```python
from build123d import *

# Parameters (mm, degrees)
SKETCH_1_R          = 2.5
EXTRUDE_1_DEPTH     = 2
SKETCH_2_R          = 1.5
EXTRUDE_2_DEPTH     = 33
FILLET_2_R          = 0.3
CUT_EXTRUDE_1_DEPTH = 1
FILLET_1_R          = 0.1


with BuildPart() as part:
    # Эскиз1 → Бобышка-Вытянуть1 (new body)
    with BuildSketch(Plane.XY):
        Circle(SKETCH_1_R)
    extrude(amount=EXTRUDE_1_DEPTH)

    # Эскиз2 → Бобышка-Вытянуть2 (add)
    with BuildSketch(Plane(origin=(0, 0, 0), x_dir=(-1, 0, 0), z_dir=(0, 0, -1))):
        Circle(SKETCH_2_R)
    extrude(amount=EXTRUDE_2_DEPTH)

    # Скругление2
    fillet_2_edges = [part.edges().sort_by_distance(p)[0] for p in [
        (-2.5, 0, 0),
        (-2.5, 0, 2),
    ]]
    fillet(fillet_2_edges, radius=FILLET_2_R)

    # Эскиз3 → Вырез-Вытянуть1 (cut)
    with BuildSketch(Plane.XY.offset(2)):
        Polygon((-0.45, 1.5), (0.45, 1.5), (0.45, 0.45), (1.5, 0.45), (1.5, -0.45), (0.45, -0.45), (0.45, -1.5), (-0.45, -1.5), (-0.45, -0.45), (-1.5, -0.45), (-1.5, 0.45), (-0.45, 0.45), align=None)
    extrude(amount=-CUT_EXTRUDE_1_DEPTH, mode=Mode.SUBTRACT)

    # Скругление1
    fillet_1_edges = [part.edges().sort_by_distance(p)[0] for p in [
        (1.5, 0, 0),
    ]]
    fillet(fillet_1_edges, radius=FILLET_1_R)


solid = part.part
```
Input: part model. Units: mm. Frame: model coordinates. A direction names the side the tool comes from. Round coordinates to 2 decimals unless told otherwise and drop trailing zeros. Loops run counter-clockwise (first coordinate to the right, second up) from the corner with the lowest first, then second, coordinate; pieces in that order, holes last. Notation, with made-up numbers: M -37.5,33.25 L 7.5,33.25 A14 ccw 7.5,60.25 Z; hole C 20.5,21 d6. An arc over 180 degrees is marked long. Answer in a Markdown table with one row per item. Add a question column.
1. Mould query, pull axis X, two halves, no side actions, for faces 4 (the face through (1.5, 0.07, -16.32)), 5 (the face through (-1, 1, 2)), 6 (the face through (0, -1.5, 1.5)). Classes: released by +X, released by -X, zero draft, split by the parting line, or undercut.
2. Set-up query: faces 1 (the face through (-1.5, 0, 1.5)), 2 (the face through (0, -2, 0)), 3 (the face through (0, 0, -33)). Return all of +Z, -Z, +X, -X, +Y, -Y with unobstructed straight access to the full face (end or side cutting, diameter ignored); none if empty.
3. Ray query, probe 1 along Z at (x, y) = (0.5, 0.1); probe 2 along Z at (x, y) = (2.1, 0.8); probe 3 along Y at (x, z) = (0.05, -18). Return the intervals inside material, ascending.
4. Contact query for flat-ended pins moving along their axis: pin 1 (2 mm diameter, centred on x = 1.5, z = -10, fed in from +Y); pin 2 (1.1 mm diameter, centred on x = -1, z = 1.5, fed in from -Y); pin 3 (0.8 mm diameter, centred on y = -1, z = 1.5, fed in from +X). Output: stop coordinate, or through.
5. Section A-A (y = 0). Output: boundary loops of the cut face in (x, z).
6. Section C-C (z = -20). Output: boundary loops of the cut face in (x, y), and give its area (3 significant figures).
Values follow:
| question | item | result |
|---|---|---|
| 1 | face 4 | split by the parting line |
| 1 | face 5 | zero draft |
| 1 | face 6 | undercut |
| 2 | face 1 | +Z |
| 2 | face 2 | -Z |
| 2 | face 3 | -Z, +X, -X, +Y, -Y |
| 3 | probe 1 | -33 to 1 |
| 3 | probe 2 | 0 to 2 |
| 3 | probe 3 | -1.5 to 1.5 |
| 4 | pin 1 | y = 1.41 |
| 4 | pin 2 | y = -2.46 |
| 4 | pin 3 | x = 2.43 |
| 5 | outline | M -2.5,0.3 A0.3 ccw -2.2,0 L -1.6,0 A0.1 cw -1.5,-0.1 L -1.5,-33 L 1.5,-33 L 1.5,-0.1 A0.1 cw 1.6,0 L 2.2,0 A0.3 ccw 2.5,0.3 L 2.5,1.7 A0.3 ccw 2.2,2 L 1.5,2 L 1.5,1 L -1.5,1 L -1.5,2 L -2.2,2 A0.3 ccw -2.5,1.7 Z |
| 6 | outline | C 0,0 d3 |
| 6 | area | 7.07 mm^2 |
